Geometry: see drawing. Coordinates: mm, zero at the bounding-box minimum. A direction names the side the tool comes from. Give positions to 0.01 mm unless a question says otherwise; leave off trailing zeros. Loops run counter-clockwise (first coordinate to the right, second up) from the corner with the lowest first, then second, coordinate; pieces in that order, holes last. Notation, with made-up numbers: (21, 22) -> (30, 22) arc R24 cw to (30, 44) -> close; hole circle Ø7 at (63.25, 41). An arc over 180 degrees is marked (long way). Return JSON: item names as keys, results as strings. Group by question number.
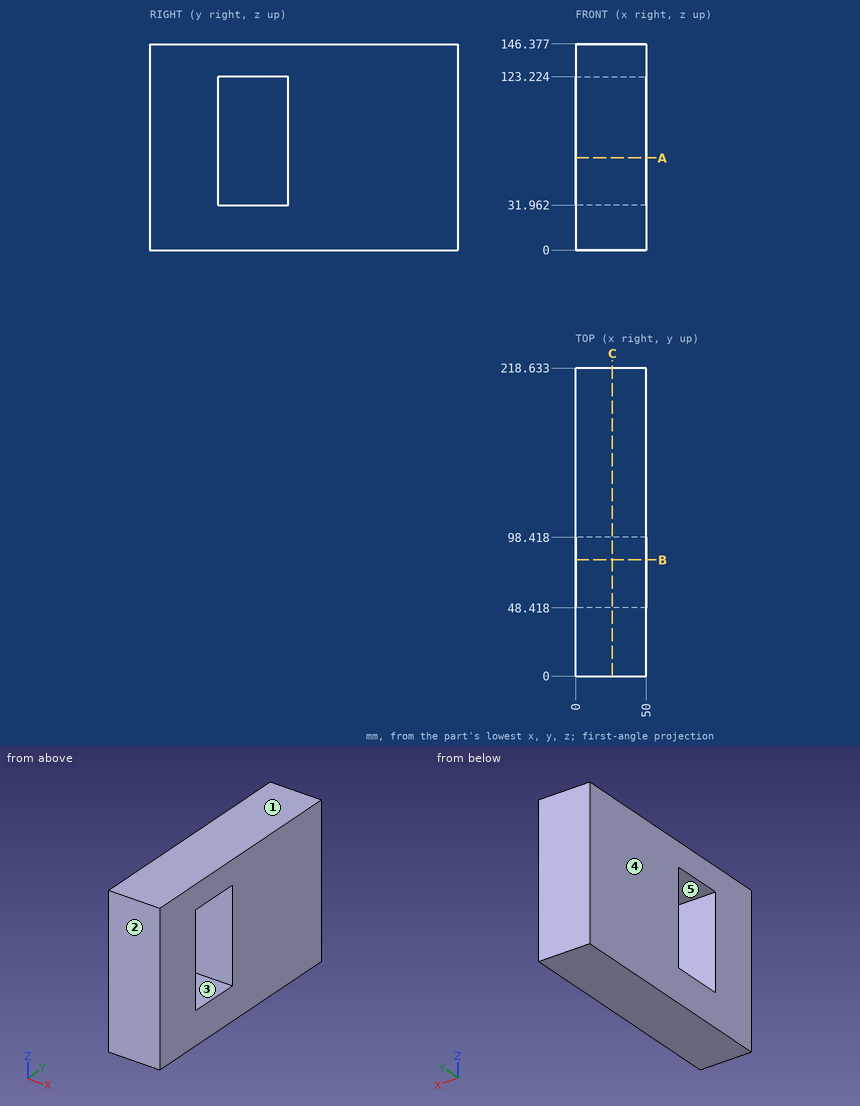
1) Reachability of the marked faces 4 and 5 from +Z, -Z, +X, -X, +Y, -Y: full face, straight path, thin tool, end or side. Return the list, or none.
2) Material intervals for line 1 (Y direction, x = 23.5, z = 76); line 2 (Z direction, x = 14, y = 54.5), sorted ascending.
3) Cut plane B-B on y = 82.5. Return loops of the section in (x, z).
4) Mould query, pull axis Z, two halves, no side actions, for the marked faces 1, 2 and 3. Classes: released by +Z, released by -Z, zero draft, split by the parting line, or undercut.
5) Cut plane C-C on x = 26. Return loops of the section in (y, z), then the cut area to 3 significant figures.
6) Cut plane A-A on z = 65.5. Return loops of the section in (x, y).
Calculated:
{
 "1": {"face 4": "+Z, -Z, -X, +Y, -Y", "face 5": "+X, -X"},
 "2": {"line 1": "0 to 48.42, 98.42 to 218.63", "line 2": "0 to 31.96, 123.22 to 146.38"},
 "3": {"outline": "(0, 0) -> (50, 0) -> (50, 31.96) -> (0, 31.96) -> close; (0, 123.22) -> (50, 123.22) -> (50, 146.38) -> (0, 146.38) -> close"},
 "4": {"face 1": "released by +Z", "face 2": "zero draft", "face 3": "undercut"},
 "5": {"outline": "(0, 0) -> (218.63, 0) -> (218.63, 146.38) -> (0, 146.38) -> close; hole (48.42, 31.96) -> (98.42, 31.96) -> (98.42, 123.22) -> (48.42, 123.22) -> close", "area": "27,400 mm2"},
 "6": {"outline": "(0, 0) -> (50, 0) -> (50, 48.42) -> (0, 48.42) -> close; (0, 98.42) -> (50, 98.42) -> (50, 218.63) -> (0, 218.63) -> close"}
}
